The listing builds one solid part. Answer for the finished solid, in the listing's coordinates (mm). Coordinates: 2 decimals unless noted, no trailing zeros. Loops run counter-clockwise (first coordinate to the right, second up) from the corner with the lowest first, then second, coordinate; pieces in that order, holes last. Notation, with made-up numbers: (43.25, -32.5) - (77.25, -32.5) arc R34 ccw to (77.25, 1.5) - close; hole circle Ø7 at (73.5, -35.75). An arc over 180 degrees is marked (long way). Write each question's results on one line, items separated by ' | '. Start each with the question number.
(1) Find section C-C on z = 3.95. Determine the outline of the cut face in (x, y).
(2) Consider line 1 (X direction, y = 13, z = 2.05); line 2 (Y direction, x = 16, z = 3.25); line 3 (Z direction, x = -9.5, y = -28). Determine where each line is inside the solid, lowest interval first. Write a range as from..to.
(3) Determine the mould class of faces 1 (the flat face through (-1, 1, 2)), 2 (the flat face through (-1, 1, 0)) for opening direction X: released by +X, released by -X, zero draft, split by the parting line, or undercut.
(4) Find section A-A on y = -8. Determine the outline of the cut face in (x, z), then the cut area to 3 significant figures.
(5) Given pin 1 Ø6 at (x, y) = (-72, 41) entering from +Z, flat-ended and moving along its own axis, determine where the tip first touches the part or whether it passes through.
from build123d import *

# Parameters (mm, degrees)
F0_W     = 182
F0_H     = 182
F1_DEPTH = 2
F0_W_2   = 192
F0_H_2   = 192
F2_DEPTH = 5
F3_R     = 2


with BuildPart() as f1:
    # F0 (on Top) → F1 (new body)
    with BuildSketch(Plane.XY):
        Rectangle(F0_W, F0_H)
    extrude(amount=F1_DEPTH)

    # F0 (on Top) → F2 (join)
    with BuildSketch(Plane.XY):
        Rectangle(F0_W_2, F0_H_2)
        Rectangle(F0_W, F0_H, mode=Mode.SUBTRACT)
    extrude(amount=F2_DEPTH)

    # F3
    f3_edges = [f1.edges().sort_by_distance(p)[0] for p in [
        (-96, -96, 2.5),
        (96, -96, 2.5),
        (0, -96, 0),
        (0, -96, 5),
        (96, 96, 2.5),
        (96, 0, 0),
        (96, 0, 5),
        (-96, 96, 2.5),
        (0, 96, 0),
        (0, 96, 5),
        (-96, 0, 0),
        (-96, 0, 5),
        (0, 91, 5),
        (91, 0, 5),
        (0, -91, 5),
        (-91, 0, 5),
    ]]
    fillet(f3_edges, radius=F3_R)


solid = f1.part
Values:
1) outline: (-95.76, -94) arc R1.76 ccw to (-94, -95.76) - (94, -95.76) arc R1.76 ccw to (95.76, -94) - (95.76, 94) arc R1.76 ccw to (94, 95.76) - (-94, 95.76) arc R1.76 ccw to (-95.76, 94) - close; hole (-91.24, -91.24) - (91.24, -91.24) - (91.24, 91.24) - (-91.24, 91.24) - close
2) line 1: x = -96..-91, 91..96 | line 2: y = -95.98..-91.02, 91.02..95.98 | line 3: z = 0..2
3) face 1: undercut | face 2: zero draft
4) outline: (-96, 2) arc R2 ccw to (-94, 0) - (94, 0) arc R2 ccw to (96, 2) - (96, 3) arc R2 ccw to (94, 5) - (93, 5) arc R2 ccw to (91, 3) - (91, 2) - (-91, 2) - (-91, 3) arc R2 ccw to (-93, 5) - (-94, 5) arc R2 ccw to (-96, 3) - close | area: 409 mm²
5) pin 1: stops at z = 2
